Verification items for the finished model (mm, model axes). A direction names the side the tool comes from. Give positions to 0.01 mm unless a question says otherwise; leave off trailing zeros. Order: outer loops, then holes, each group sorted by start corner. A loop starts at its lowest first (then second) coordinate and runs counter-clockwise, first axis right, second up.
from build123d import *

# Parameters (mm, degrees)
ESQUISSE1_W                     = 186
ESQUISSE1_H                     = 51
BOSS_EXTRU_1_DEPTH              = 35
ESQUISSE7_W                     = 13
ESQUISSE7_H                     = 13
ENL_V_MAT_EXTRU_5_DEPTH         = 91
R_P_TITION_LIN_AIRE5_COUNT      = 3
R_P_TITION_LIN_AIRE5_PITCH      = 16
ESQUISSE8_W                     = 13
ESQUISSE8_H                     = 13
ENL_V_MAT_EXTRU_6_DEPTH         = 103
R_P_TITION_LIN_AIRE6_COUNT      = 3
R_P_TITION_LIN_AIRE6_PITCH      = 16
R_P_TITION_LIN_AIRE6_COUNT_DIR2 = 3
R_P_TITION_LIN_AIRE6_PITCH_DIR2 = 16
ESQUISSE9_W                     = 13
ESQUISSE9_H                     = 13
ENL_V_MAT_EXTRU_7_DEPTH         = 77
R_P_TITION_LIN_AIRE7_COUNT      = 3
R_P_TITION_LIN_AIRE7_PITCH      = 16
R_P_TITION_LIN_AIRE7_COUNT_DIR2 = 2
R_P_TITION_LIN_AIRE7_PITCH_DIR2 = 16
ESQUISSE10_W                    = 13
ESQUISSE10_H                    = 13
ENL_V_MAT_EXTRU_8_DEPTH         = 78
R_P_TITION_LIN_AIRE8_COUNT      = 3
R_P_TITION_LIN_AIRE8_PITCH      = 16
R_P_TITION_LIN_AIRE8_COUNT_DIR2 = 3
R_P_TITION_LIN_AIRE8_PITCH_DIR2 = 16
ESQUISSE14_W                    = 10
ESQUISSE14_H                    = 5
BOSS_EXTRU_3_DEPTH              = 7
ESQUISSE25_W                    = 186
ESQUISSE25_H                    = 35
BOSS_EXTRU_7_DEPTH              = 7
ESQUISSE18_W                    = 186
ESQUISSE18_H                    = 35
BOSS_EXTRU_5_DEPTH              = 7
ESQUISSE16_W                    = 3.3
ESQUISSE16_H                    = 55
ENL_V_MAT_EXTRU_11_DEPTH        = 184
ESQUISSE15_R                    = 1
ENL_V_MAT_EXTRU_10_DEPTH        = 7
ESQUISSE24_W                    = 10
ESQUISSE24_H                    = 2
ENL_V_MAT_EXTRU_12_DEPTH        = 1
ESQUISSE19_W                    = 186
ESQUISSE19_H                    = 1
ESQUISSE19_W_2                  = 1
ESQUISSE19_H_2                  = 63
BOSS_EXTRU_8_DEPTH              = 30
ESQUISSE26_R                    = 1.75
ENL_V_MAT_EXTRU_14_DEPTH        = 30
ESQUISSE27_R                    = 1.75
ENL_V_MAT_EXTRU_20_DEPTH        = 198.952014387


with BuildPart() as part:
    # Esquisse1 → Boss.-Extru.1 (new body)
    with BuildSketch(Plane.XY):
        with Locations((0, -25.5)):
            Rectangle(ESQUISSE1_W, ESQUISSE1_H)
    extrude(amount=BOSS_EXTRU_1_DEPTH)

    # Esquisse7 → Enlèv. mat.-Extru.5 (cut)
    with BuildSketch(Plane.XY.offset(35)):
        with Locations((-83.5, -9.5)):
            Rectangle(ESQUISSE7_W, ESQUISSE7_H)
    enl_v_mat_extru_5 = extrude(amount=-ENL_V_MAT_EXTRU_5_DEPTH, mode=Mode.SUBTRACT)

    # Répétition linéaire5: Enlèv. mat.-Extru.5 ×3
    with Locations(*[(0, -i * R_P_TITION_LIN_AIRE5_PITCH, 0) for i in range(1, R_P_TITION_LIN_AIRE5_COUNT)]):
        add(enl_v_mat_extru_5, mode=Mode.SUBTRACT)

    # Esquisse8 → Enlèv. mat.-Extru.6 (cut)
    with BuildSketch(Plane.XY.offset(35)):
        with Locations((-54.5, -9.5)):
            Rectangle(ESQUISSE8_W, ESQUISSE8_H)
    enl_v_mat_extru_6 = extrude(amount=-ENL_V_MAT_EXTRU_6_DEPTH, mode=Mode.SUBTRACT)

    # Répétition linéaire6: Enl_v. mat.-Extru.6 3 × 3
    with Locations(*[(j * R_P_TITION_LIN_AIRE6_PITCH_DIR2, -i * R_P_TITION_LIN_AIRE6_PITCH, 0) for i in range(R_P_TITION_LIN_AIRE6_COUNT) for j in range(R_P_TITION_LIN_AIRE6_COUNT_DIR2) if (i, j) != (0, 0)]):
        add(enl_v_mat_extru_6, mode=Mode.SUBTRACT)

    # Esquisse9 → Enlèv. mat.-Extru.7 (cut)
    with BuildSketch(Plane.XY.offset(35)):
        with Locations((6.5, -9.5)):
            Rectangle(ESQUISSE9_W, ESQUISSE9_H)
    enl_v_mat_extru_7 = extrude(amount=-ENL_V_MAT_EXTRU_7_DEPTH, mode=Mode.SUBTRACT)

    # Répétition linéaire7: Enl_v. mat.-Extru.7 3 × 2
    with Locations(*[(j * R_P_TITION_LIN_AIRE7_PITCH_DIR2, -i * R_P_TITION_LIN_AIRE7_PITCH, 0) for i in range(R_P_TITION_LIN_AIRE7_COUNT) for j in range(R_P_TITION_LIN_AIRE7_COUNT_DIR2) if (i, j) != (0, 0)]):
        add(enl_v_mat_extru_7, mode=Mode.SUBTRACT)

    # Esquisse10 → Enlèv. mat.-Extru.8 (cut)
    with BuildSketch(Plane.XY.offset(35)):
        with Locations((51.5, -9.5)):
            Rectangle(ESQUISSE10_W, ESQUISSE10_H)
    enl_v_mat_extru_8 = extrude(amount=-ENL_V_MAT_EXTRU_8_DEPTH, mode=Mode.SUBTRACT)

    # Répétition linéaire8: Enl_v. mat.-Extru.8 3 × 3
    with Locations(*[(i * R_P_TITION_LIN_AIRE8_PITCH, -j * R_P_TITION_LIN_AIRE8_PITCH_DIR2, 0) for i in range(R_P_TITION_LIN_AIRE8_COUNT) for j in range(R_P_TITION_LIN_AIRE8_COUNT_DIR2) if (i, j) != (0, 0)]):
        add(enl_v_mat_extru_8, mode=Mode.SUBTRACT)

    # Esquisse14 → Boss.-Extru.3 (add)
    with BuildSketch(Plane.XZ.offset(51)):
        with Locations((-7.663083533, 2.5)):
            Rectangle(ESQUISSE14_W, ESQUISSE14_H)
    extrude(amount=BOSS_EXTRU_3_DEPTH)

    # Esquisse25 → Boss.-Extru.7 (add)
    with BuildSketch(Plane(origin=(0, 0, 0), x_dir=(1, 0, 0), z_dir=(0, 1, 0))):
        with Locations((0, -17.5)):
            Rectangle(ESQUISSE25_W, ESQUISSE25_H)
    extrude(amount=BOSS_EXTRU_7_DEPTH)

    # Esquisse18 → Boss.-Extru.5 (add)
    with BuildSketch(Plane.XZ.offset(51)):
        with Locations((0, 17.5)):
            Rectangle(ESQUISSE18_W, ESQUISSE18_H)
    extrude(amount=BOSS_EXTRU_5_DEPTH)

    # Esquisse16 → Enlèv. mat.-Extru.11 (cut)
    with BuildSketch(Plane.ZY.offset(93)):
        with Locations((31.65, -25.5)):
            Rectangle(ESQUISSE16_W, ESQUISSE16_H)
    extrude(amount=-ENL_V_MAT_EXTRU_11_DEPTH, mode=Mode.SUBTRACT)

    # Esquisse15 → Enlèv. mat.-Extru.10 (cut)
    with BuildSketch(Plane(origin=(0, 0, 0), x_dir=(-1, 0, 0), z_dir=(0, 0, -1))):
        with Locations((8.482305804, -42.446555864)):
            Circle(ESQUISSE15_R)
        with Locations((8.482305804, -9.749028666)):
            Circle(ESQUISSE15_R)
        with Locations((68.823038652, -42.446555864)):
            Circle(ESQUISSE15_R)
        with Locations((68.823038652, -9.749028666)):
            Circle(ESQUISSE15_R)
        with Locations((-37.13548256, -42.446555864)):
            Circle(ESQUISSE15_R)
        with Locations((-39.215855023, -11.260648292)):
            Circle(ESQUISSE15_R)
    extrude(amount=-ENL_V_MAT_EXTRU_10_DEPTH, mode=Mode.SUBTRACT)

    # Esquisse24 → Enlèv. mat.-Extru.12 (cut)
    with BuildSketch(Plane(origin=(0, 0, 0), x_dir=(-1, 0, 0), z_dir=(0, 0, -1))):
        with Locations((83.5, -49)):
            Rectangle(ESQUISSE24_W, ESQUISSE24_H)
        with Locations((54.5, -49)):
            Rectangle(ESQUISSE24_W, ESQUISSE24_H)
        with Locations((38.5, -49)):
            Rectangle(ESQUISSE24_W, ESQUISSE24_H)
        with Locations((22.5, -49)):
            Rectangle(ESQUISSE24_W, ESQUISSE24_H)
        with Locations((-6.5, -49)):
            Rectangle(ESQUISSE24_W, ESQUISSE24_H)
        with Locations((-22.5, -49)):
            Rectangle(ESQUISSE24_W, ESQUISSE24_H)
        with Locations((-51.5, -49)):
            Rectangle(ESQUISSE24_W, ESQUISSE24_H)
        with Locations((-67.5, -49)):
            Rectangle(ESQUISSE24_W, ESQUISSE24_H)
        with Locations((-83.5, -49)):
            Rectangle(ESQUISSE24_W, ESQUISSE24_H)
        with Locations((-83.5, -2)):
            Rectangle(ESQUISSE24_W, ESQUISSE24_H)
        with Locations((-67.5, -2)):
            Rectangle(ESQUISSE24_W, ESQUISSE24_H)
        with Locations((-51.5, -2)):
            Rectangle(ESQUISSE24_W, ESQUISSE24_H)
        with Locations((-22.5, -2)):
            Rectangle(ESQUISSE24_W, ESQUISSE24_H)
        with Locations((-6.5, -2)):
            Rectangle(ESQUISSE24_W, ESQUISSE24_H)
        with Locations((22.5, -2)):
            Rectangle(ESQUISSE24_W, ESQUISSE24_H)
        with Locations((38.5, -2)):
            Rectangle(ESQUISSE24_W, ESQUISSE24_H)
        with Locations((54.5, -2)):
            Rectangle(ESQUISSE24_W, ESQUISSE24_H)
        with Locations((83.5, -2)):
            Rectangle(ESQUISSE24_W, ESQUISSE24_H)
    extrude(amount=-ENL_V_MAT_EXTRU_12_DEPTH, mode=Mode.SUBTRACT)

    # Esquisse19 → Boss.-Extru.8 (add)
    with BuildSketch(Plane(origin=(0, 0, 0), x_dir=(-1, 0, 0), z_dir=(0, 0, -1))):
        with Locations((0, -57.5)):
            Rectangle(ESQUISSE19_W, ESQUISSE19_H)
        with Locations((92.5, -25.5)):
            Rectangle(ESQUISSE19_W_2, ESQUISSE19_H_2)
        with Locations((0, 6.5)):
            Rectangle(ESQUISSE19_W, ESQUISSE19_H)
        with Locations((-92.5, -25.5)):
            Rectangle(ESQUISSE19_W_2, ESQUISSE19_H_2)
    extrude(amount=BOSS_EXTRU_8_DEPTH)

    # Esquisse26 → Enlèv. mat.-Extru.14 (cut)
    with BuildSketch(Plane.ZY.offset(93)):
        with Locations((-13.75, -25.5)):
            Circle(ESQUISSE26_R)
    extrude(amount=-ENL_V_MAT_EXTRU_14_DEPTH, mode=Mode.SUBTRACT)

    # Esquisse27 → Enlèv. mat.-Extru.20 (cut, through all)
    # profile 1 of 2: a face of its own
    with BuildSketch(Plane.ZY.offset(93)):
        Polygon((30, -53), (30, 2), (20, 2), (20, 7), (-30, 7), (-30, -58), (20, -58), (20, -53), align=None)
        with Locations((-13.75, -25.5)):
            Circle(ESQUISSE27_R, mode=Mode.SUBTRACT)
    # profile 2 of 2: a face of its own
    with BuildSketch(Plane.ZY.offset(93)):
        with Locations((-13.75, -25.5)):
            Circle(ESQUISSE27_R)
    extrude(amount=-ENL_V_MAT_EXTRU_20_DEPTH, mode=Mode.SUBTRACT)


solid = part.part
(1) Section check C-C, the plane y = -10. Give the number of separate pieces and of enclosed holes in the cut face, then the cut area to 3 significant figures.
Solved:
separate pieces: 10
enclosed holes: 0
area: 124 mm2
(2) Set-up check for faces 4 (the flat face through (-1, 2, 27)), 5 (the flat face through (-93, -26, 34)): record each of +Z, -Z, +X, -X, +Y, -Y from which the full face is reachable in a straight line by a thin tool's end or side.
Solved:
face 4: -Z, -X
face 5: +Z, -Z, -X, +Y, -Y
(3) Section check A-A, the plane z = 25.25. Enter the section's corners in (x, y).
Solved:
outline: (-93, -58) - (93, -58) - (93, -53) - (-93, -53) - close; (-93, 2) - (93, 2) - (93, 7) - (-93, 7) - close
(4) Section check B-B, the plane x = 63. Enter the section's corners in (y, z), then the cut area to 3 significant figures.
Solved:
outline: (-58, 20) - (-53, 20) - (-53, 33.3) - (-48, 33.3) - (-48, 35) - (-58, 35) - close; (-35, 33.3) - (-32, 33.3) - (-32, 35) - (-35, 35) - close; (-19, 33.3) - (-16, 33.3) - (-16, 35) - (-19, 35) - close; (-3, 33.3) - (2, 33.3) - (2, 20) - (7, 20) - (7, 35) - (-3, 35) - close
area: 177 mm2
(5) Release check for a two-part mould opening along Y. For faces 1 (the flat face through (-1, 4, 20)), 2 (the flat face through (1, 7, 28)), 3 (the flat face through (91, -25, 32)) record: pulls with the +Y half, pulls with the -Y half, needs draft (parallel to the pull), parting line crosses it, or undercut.
Solved:
face 1: needs draft
face 2: pulls with the +Y half
face 3: undercut
(6) Scan lines: line 1 (Y direction, x = -59, z = 34); line 2 (Y direction, x = 72.5, z = 21); line 3 (Z direction, x = -3, y = -0.5). Record each from-to range of solid material in increasing order.
Solved:
line 1: y = -58 to -48, -35 to -32, -19 to -16, -3 to 7
line 2: y = -58 to -53, 2 to 7
line 3: z = 33.3 to 35
(7) Go/stop test with flat-tipped pins: pin 1 (3 mm diameter, centred on x = -1.5, y = -19, fed in from -Z); pin 2 (1 mm diameter, centred on y = -34.5, z = 32.5, fed in from -X); pin 3 (0.6 mm diameter, centred on x = 92, y = -25.5, fed in from -Z). Record where each tip stops, or that it passes through.
Solved:
pin 1: stops at z = 33.3
pin 2: stops at x = 91
pin 3: stops at z = 30
